Check sheet for the modelled part. Datum: model origin and axes. Units: mm. Give positions to 0.01 mm unless a question says otherwise; leave off trailing zeros. Loops run counter-clockwise (first coordinate to the right, second up) from the corner with the lowest first, then second, coordinate; pieces in that order, holes last. Notation, with made-up numbers: (20, -40) - (38, -40) arc R23 ccw to (38, -21) - close; hole circle Ø10 at (9.5, -20.5). An arc over 180 degrees is marked (long way). Use CSV: the item, a comma, the result in double quotes.
from build123d import *

# Parameters (mm, degrees)
SKETCH1_W           = 56
SKETCH1_H           = 71
BOSS_EXTRUDE1_DEPTH = 8
FILLET1_R           = 2
SKETCH2_R           = 2
SKETCH2_R_2         = 12.5
CUT_EXTRUDE1_DEPTH  = 91.779953734


with BuildPart() as part:
    # Sketch1 → Boss-Extrude1 (new body)
    with BuildSketch(Plane(origin=(0, 0, 0), x_dir=(1, 0, 0), z_dir=(0, 1, 0))):
        with Locations((28, 35.5)):
            Rectangle(SKETCH1_W, SKETCH1_H)
    extrude(amount=BOSS_EXTRUDE1_DEPTH)

    # Fillet1
    fillet1_edges = [part.edges().sort_by_distance(p)[0] for p in [
        (0, 4, -71),
        (56, 4, -71),
        (56, 4, 0),
        (0, 4, 0),
    ]]
    fillet(fillet1_edges, radius=FILLET1_R)

    # Sketch2 → Cut-Extrude1 (cut, through all)
    with BuildSketch(Plane(origin=(0, 8, 0), x_dir=(1, 0, 0), z_dir=(0, 1, 0))):
        with Locations(Location((4.5, 66.5, 0), (0, 0, 270))):
            Circle(SKETCH2_R)
        with Locations(Location((51.5, 66.5, 0), (0, 0, 270))):
            Circle(SKETCH2_R)
        with Locations(Location((51.5, 19.5, 0), (0, 0, 270))):
            Circle(SKETCH2_R)
        with Locations(Location((4.5, 19.5, 0), (0, 0, 270))):
            Circle(SKETCH2_R)
        with Locations(Location((28, 43, 0), (0, 0, 270))):
            Circle(SKETCH2_R_2)
    extrude(amount=-CUT_EXTRUDE1_DEPTH, mode=Mode.SUBTRACT)


solid = part.part
1. Sectioned sample at A-A, the plane z = -19.5. Record the boundary of the cut face in (x, y), and give its area (3 significant figures).
Completed:
outline,"(0, 0) - (2.5, 0) - (2.5, 8) - (0, 8) - close; (6.5, 0) - (49.5, 0) - (49.5, 8) - (6.5, 8) - close; (53.5, 0) - (56, 0) - (56, 8) - (53.5, 8) - close"
area,"384 mm²"
2. Scan lines: line 1 along X through (y, z) = (4, -19.5); line 2 along Z through (x, y) = (3, 7.75); line 3 along Z through (x, y) = (5.5, 3.25). Record each from-to range of solid material in increasing order.
Completed:
line 1,"x = 0 to 2.5, 6.5 to 49.5, 53.5 to 56"
line 2,"z = -71 to -67.82, -65.18 to -20.82, -18.18 to 0"
line 3,"z = -71 to -68.23, -64.77 to -21.23, -17.77 to 0"
3. Sectioned sample at C-C, the plane x = 4.5. Record the boundary of the cut face in (y, z).
Completed:
outline,"(0, -71) - (8, -71) - (8, -68.5) - (0, -68.5) - close; (0, -64.5) - (8, -64.5) - (8, -21.5) - (0, -21.5) - close; (0, -17.5) - (8, -17.5) - (8, 0) - (0, 0) - close"
4. Go/stop test with a flat-tipped pin: pin 1 Ø6.5 at (x, z) = (51.5, -19.5) entering from +Y. Record where the tip stops, or that it passes through.
Completed:
pin 1,"stops at y = 8"
5. Release check for a two-part mould opening along X. For faces 1 (the face through (2.726, 4.056, -18.577)), 2 (the face through (20.394, 4.056, -52.92)), 3 (the face through (28, 8, -28)), 4 (the face through (55.43, 4.06, -70.4)) record: released by +X, released by -X, zero draft, split by the parting line, or undercut.
Completed:
face 1,"undercut"
face 2,"undercut"
face 3,"zero draft"
face 4,"released by +X"
6. Sectioned sample at B-B, the plane y = 1. Record the boundary of the cut face in (x, z).
Completed:
outline,"(0, -69) arc R2 ccw to (2, -71) - (54, -71) arc R2 ccw to (56, -69) - (56, -2) arc R2 ccw to (54, 0) - (2, 0) arc R2 ccw to (0, -2) - close; hole circle Ø4 at (4.5, -66.5); hole circle Ø4 at (4.5, -19.5); hole circle Ø25 at (28, -43); hole circle Ø4 at (51.5, -66.5); hole circle Ø4 at (51.5, -19.5)"
7. Sectioned sample at D-D, the plane x = 28. Record the boundary of the cut face in (y, z).
Completed:
outline,"(0, -71) - (8, -71) - (8, -55.5) - (0, -55.5) - close; (0, -30.5) - (8, -30.5) - (8, 0) - (0, 0) - close"
